Verification items for the finished model (mm, model axes). A direction names the side the tool comes from. Round coordinates to 2 decimals unless told otherwise and drop trailing zeros. Write each loop counter-clockwise with the first axis right and the second up, starting at its lowest first coordinate (ties: lowest second). Pieces come first, ordered by that corner, then holes. Notation, with made-up numbers: (36, -1) - (92, -1) arc R23 ccw to (92, 20) - close; hole circle Ø8 at (-12.5, 86). An arc over 180 degrees is marked (long way). Answer as a JSON object with one key per item and string values.
```python
from build123d import *

# Parameters (mm, degrees)
BOSS_EXTRUDE1_DEPTH = 15
CUT_EXTRUDE1_REACH  = 35.839
SKETCH5_R           = 1.7
CHAMFER1_SIZE       = 3


with BuildPart() as part:
    # Sketch2 → Revolve1 (revolve)
    with BuildSketch(Plane.XY, mode=Mode.PRIVATE) as revolve1_sk:
        Polygon((0, 0), (-20, 0), (-20, 20), (-17, 20), (-17, 2), (0, 2), align=None)
    revolve(revolve1_sk.sketch.rotate(Axis((0, 0, 0), (0, 1, 0)), 270), axis=Axis((0, 0, 0), (0, 1, 0)))

    # Sketch3 → Boss-Extrude1 (add)
    with BuildSketch(Plane(origin=(0, 20, 0), x_dir=(1, 0, 0), z_dir=(0, 1, 0))):
        with BuildLine():
            ThreePointArc((-1.25, 19.960899278), (0, 20.52), (1.25, 19.960899278))
            ThreePointArc((1.25, 19.960899278), (0, 20), (-1.25, 19.960899278))
        make_face()
        with BuildLine():
            ThreePointArc((16.661645857, 11.062981394), (17.320508076, 10), (17.911645857, 8.897917884))
            ThreePointArc((17.911645857, 8.897917884), (17.770841286, 10.26), (16.661645857, 11.062981394))
        make_face()
        with BuildLine():
            ThreePointArc((17.911645857, -8.897917884), (17.320508076, -10), (16.661645857, -11.062981394))
            ThreePointArc((16.661645857, -11.062981394), (17.770841286, -10.26), (17.911645857, -8.897917884))
        make_face()
        with BuildLine():
            ThreePointArc((1.25, -19.960899278), (0, -20), (-1.25, -19.960899278))
            ThreePointArc((-1.25, -19.960899278), (0, -20.52), (1.25, -19.960899278))
        make_face()
        with BuildLine():
            ThreePointArc((-16.661645857, -11.062981394), (-17.320508076, -10), (-17.911645857, -8.897917884))
            ThreePointArc((-17.911645857, -8.897917884), (-17.770841286, -10.26), (-16.661645857, -11.062981394))
        make_face()
        with BuildLine():
            ThreePointArc((-17.911645857, 8.897917884), (-17.320508076, 10), (-16.661645857, 11.062981394))
            ThreePointArc((-16.661645857, 11.062981394), (-17.770841286, 10.26), (-17.911645857, 8.897917884))
        make_face()
    extrude(amount=-BOSS_EXTRUDE1_DEPTH)

    # Sketch4 → Cut-Revolve1 (revolve, cut)
    with BuildSketch(Plane.XY, mode=Mode.PRIVATE) as cut_revolve1_sk:
        Polygon((-21, 16.767949192), (-18.556624327, 21), (-21, 21), align=None)
    revolve(cut_revolve1_sk.sketch.rotate(Axis((0, 20, 0), (0, -1, 0)), 90), axis=Axis((0, 20, 0), (0, -1, 0)), mode=Mode.SUBTRACT)

    # Sketch5 → Cut-Extrude1 (cut, up to next)
    with BuildSketch(Plane(origin=(0, 2, 0), x_dir=(1, 0, 0), z_dir=(0, 1, 0)), mode=Mode.PRIVATE) as cut_extrude1_sk1:
        with Locations(Location((0, 9.5, 0), (0, 0, 270))):
            Circle(SKETCH5_R)
    cut_extrude1_tool1 = extrude(cut_extrude1_sk1.sketch, amount=-CUT_EXTRUDE1_REACH, mode=Mode.PRIVATE) & part.part
    # Sketch5 → Cut-Extrude1 (cut, up to next)
    with BuildSketch(Plane(origin=(0, 2, 0), x_dir=(1, 0, 0), z_dir=(0, 1, 0)), mode=Mode.PRIVATE) as cut_extrude1_sk2:
        with Locations(Location((8.227241336, -4.75, 0), (0, 0, 270))):
            Circle(SKETCH5_R)
    cut_extrude1_tool2 = extrude(cut_extrude1_sk2.sketch, amount=-CUT_EXTRUDE1_REACH, mode=Mode.PRIVATE) & part.part
    # Sketch5 → Cut-Extrude1 (cut, up to next)
    with BuildSketch(Plane(origin=(0, 2, 0), x_dir=(1, 0, 0), z_dir=(0, 1, 0)), mode=Mode.PRIVATE) as cut_extrude1_sk3:
        with Locations(Location((-8.227241336, -4.75, 0), (0, 0, 270))):
            Circle(SKETCH5_R)
    cut_extrude1_tool3 = extrude(cut_extrude1_sk3.sketch, amount=-CUT_EXTRUDE1_REACH, mode=Mode.PRIVATE) & part.part
    add(cut_extrude1_tool1.solids().sort_by_distance((0, 2, -9.5))[0], mode=Mode.SUBTRACT)
    add(cut_extrude1_tool2.solids().sort_by_distance((8.227241, 2, 4.75))[0], mode=Mode.SUBTRACT)
    add(cut_extrude1_tool3.solids().sort_by_distance((-8.227241, 2, 4.75))[0], mode=Mode.SUBTRACT)

    # Chamfer1
    chamfer1_edges = [part.edges().sort_by_distance(p)[0] for p in [
        (0, 2, 17),
    ]]
    chamfer(chamfer1_edges, length=CHAMFER1_SIZE)


solid = part.part
```
1. Go/stop test with flat-tipped pins: pin 1 (5 mm diameter, centred on y = 11, z = -12, fed in from -X); pin 2 (12 mm diameter, centred on y = 7.5, z = 16, fed in from +X); pin 3 (2 mm diameter, centred on y = 10, z = 7, fed in from +X); pin 4 (2.5 mm diameter, centred on x = -8.23, z = 4.75, fed in from -Y). Record where each tip stops, or that it passes through.
Completed:
{"pin 1": "stops at x = -17.99", "pin 2": "stops at x = 17.89", "pin 3": "stops at x = 19.08", "pin 4": "passes through"}
2. Cross-section at C-C (y = 2.75). Record the boundary of the cut face in (x, z).
Completed:
{"outline": "circle Ø40 at (0, 0); hole circle Ø29.5 at (0, 0)"}
3. Material ranges on probe 1 along X at (y, z) = (11.25, 0); probe 2 along X at (y, z) = (1, 4); probe 3 along X at (y, z) = (1.3, 4.75), recorded low to high. Write a range as from..to.
Completed:
{"probe 1": "x = -20..-17, 17..20", "probe 2": "x = -19.6..-9.75, -6.7..6.7, 9.75..19.6", "probe 3": "x = -19.43..-9.93, -6.53..6.53, 9.93..19.43"}
4. Cross-section at B-B (z = 0). Record the boundary of the cut face in (x, y), plus the area to 3 significant figures.
Completed:
{"outline": "(-20, 0) - (20, 0) - (20, 18.5) - (19.13, 20) - (17, 20) - (17, 5) - (14, 2) - (-14, 2) - (-17, 5) - (-17, 20) - (-19.13, 20) - (-20, 18.5) - close", "area": "196 mm^2"}
5. Cross-section at A-A (x = 0). Record the boundary of the cut face in (y, z), plus the area to 3 significant figures.
Completed:
{"outline": "(0, -20) - (5, -20) - (5, -20.52) - (17.6, -20.52) - (20, -19.13) - (20, -17) - (5, -17) - (2, -14) - (2, -11.2) - (0, -11.2) - close; (0, -7.8) - (2, -7.8) - (2, 14) - (5, 17) - (20, 17) - (20, 19.13) - (17.6, 20.52) - (5, 20.52) - (5, 20) - (0, 20) - close", "area": "202 mm^2"}
6. Access from +Z, -Z, +X, -X, +Y, -Y to the whole of each face (thin tool, end or side, straight path). Record for faces 1 (the face through (0, 2, 0)), 2 (the face through (-1.66, 1.01, -9.87)).
Completed:
{"face 1": "+Y", "face 2": "+Y, -Y"}
7. Mould release check, pull along X, two halves, no side actions. Record for faces 3 (the face through (17.5, 5, -10.1)), 4 (the face through (-17.76, 11.84, -10.28)), 5 (the face through (6.7, 1, 5.5)): released by +X, released by -X, zero draft, split by the parting line, or undercut.
Completed:
{"face 3": "zero draft", "face 4": "released by -X", "face 5": "undercut"}
8. Cross-section at D-D (y = 15). Record the boundary of the cut face in (x, z), plus the area to 3 significant figures.
Completed:
{"outline": "(-17.91, -8.9) arc R1.68 ccw to (-16.66, -11.06) arc R20 ccw to (-1.25, -19.96) arc R1.68 ccw to (1.25, -19.96) arc R20 ccw to (16.66, -11.06) arc R1.68 ccw to (17.91, -8.9) arc R20 ccw to (17.91, 8.9) arc R1.68 ccw to (16.66, 11.06) arc R20 ccw to (1.25, 19.96) arc R1.68 ccw to (-1.25, 19.96) arc R20 ccw to (-16.66, 11.06) arc R1.68 ccw to (-17.91, 8.9) arc R20 ccw to start; hole circle Ø34 at (0, 0)", "area": "354 mm^2"}
